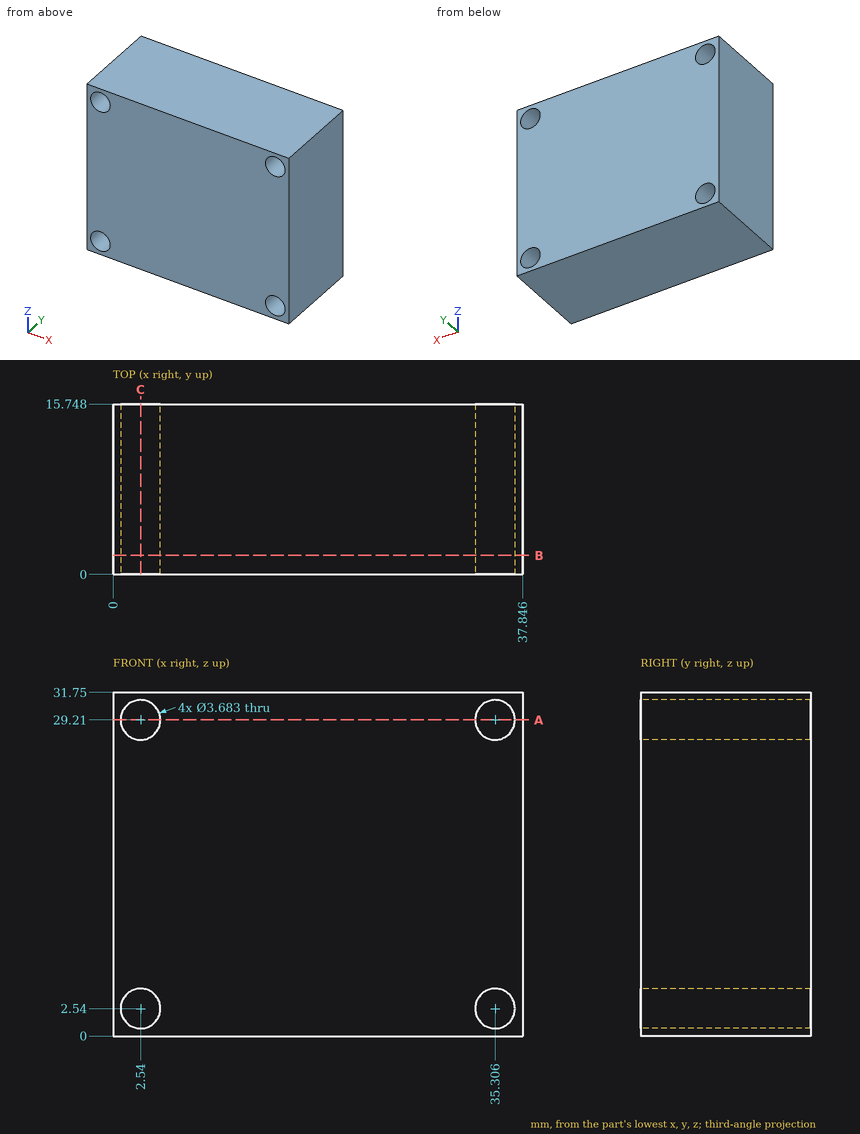
Geometry: see drawing. Coordinates: mm, zero at the bounding-box minimum. Round coordinates to 2 decimals unless told otherwise and drop trailing zeros. Order: outer loops, then holes, each group sorted by start corner. A loop starts at its lowest first (then second) coordinate and runs counter-clockwise, first axis right, second up. Notation, with made-up numbers: (-19.75, 44.5) - (4.25, 44.5) arc R13 ccw to (4.25, 55.5) - close; hole circle Ø10 at (35.25, 28). An arc over 180 degrees is marked (long way). One line per question, with ' | ' between items. Start each with the question number.
1) Cut plane A-A, the plane z = 29.21. Return the cut outline in (x, y), then the cut area to 3 significant figures.
2) Cut plane C-C, the plane x = 2.54. Return the cut outline in (y, z).
3) Ray query, probe 1 along Z at (x, y) = (2.54, 11.25); probe 2 along Z at (x, y) = (35.5, 2.25); probe 3 along X at (y, z) = (15, 3). Return the intervals inside material, ascending.
4) Cut plane B-B, the plane y = 1.75. Return the cut outline in (x, z), then the cut area to 3 significant figures.
5) Contact query for a flat-ended pin moving along its axis: P1, Ø3.5, axis at x = 2.54, z = 29.21, coming from the -Y side. Output: stop coordinate, or through.
Worked out:
1) outline: (0, 0) - (0.7, 0) - (0.7, 15.75) - (0, 15.75) - close; (4.38, 0) - (33.46, 0) - (33.46, 15.75) - (4.38, 15.75) - close; (37.15, 0) - (37.85, 0) - (37.85, 15.75) - (37.15, 15.75) - close | area: 480 mm^2
2) outline: (0, 0) - (15.75, 0) - (15.75, 0.7) - (0, 0.7) - close; (0, 4.38) - (15.75, 4.38) - (15.75, 27.37) - (0, 27.37) - close; (0, 31.05) - (15.75, 31.05) - (15.75, 31.75) - (0, 31.75) - close
3) probe 1: z = 0 to 0.7, 4.38 to 27.37, 31.05 to 31.75 | probe 2: z = 0 to 0.71, 4.37 to 27.38, 31.04 to 31.75 | probe 3: x = 0 to 0.76, 4.32 to 33.52, 37.09 to 37.85
4) outline: (0, 0) - (37.85, 0) - (37.85, 31.75) - (0, 31.75) - close; hole circle Ø3.68 at (2.54, 2.54); hole circle Ø3.68 at (2.54, 29.21); hole circle Ø3.68 at (35.31, 2.54); hole circle Ø3.68 at (35.31, 29.21) | area: 1,160 mm^2
5) P1: passes through
